```python
from build123d import *

# Parameters (mm, degrees)
F1_DEPTH = 29
F3_DEPTH = 21
F5_D     = 5
F6_D     = 5
F7_D     = 5
F7_DEPTH = 10
F7_TIP   = 1.5021515476
F9_D     = 11.2


with BuildPart() as f1:
    # F0 (on Right) → F1 (new body, symmetric)
    with BuildSketch(Plane.YZ):
        Polygon((-22.1, 20), (-25, 20), (-25, -20), (25, -20), (25, 20), (22.1, 20), (0, -2.1), align=None)
    extrude(amount=F1_DEPTH, both=True)

    # F2 (on Right) → F3 (cut, symmetric)
    with BuildSketch(Plane.YZ):
        Polygon((7, -20), (25, -20), (25, -2), align=None)
    extrude(amount=F3_DEPTH, both=True, mode=Mode.SUBTRACT)

    # F5 (through all)
    with Locations(Plane(origin=(-29, 0, 0), x_dir=(0, -1, 0), z_dir=(-1, 0, 0))):
        with Locations((-19, -14), (19, -14)):
            Hole(F5_D / 2)

    # F6 (through all)
    with Locations(Plane(origin=(-29, 0, 0), x_dir=(0, -1, 0), z_dir=(-1, 0, 0))):
        with Locations((-19, 6), (19, 6)):
            Hole(F6_D / 2)

    # F7
    with Locations(Plane(origin=(-29, 0, 0), x_dir=(0, -1, 0), z_dir=(-1, 0, 0))):
        with Locations((-19, -4), (19, -4)):
            Hole(F7_D / 2, depth=F7_DEPTH)
            with Locations((0, 0, -(F7_DEPTH + F7_TIP / 2))):  # 118° drill point
                Cone(0, F7_D / 2, F7_TIP, mode=Mode.SUBTRACT)

    # F9 (through all)
    with Locations(Plane(origin=(0, 13.5, -13.5), x_dir=(-1, 0, 0), z_dir=(0, 0.7071067812, -0.7071067812))):
        with Locations((-10.5, 4.5150757595), (10.5, 4.5150757595)):
            Hole(F9_D / 2)


solid = f1.part
```
Could you check a few things on this model? Use its own coordinates, in mm. A direction names the side the tool comes from. Coordinates: 2 decimals unless noted, no trailing zeros. Write each loop counter-clockwise with the first axis right and the second up, starting at its lowest first coordinate (ties: lowest second). Pieces come first, ordered by that corner, then holes. Notation, with made-up numbers: (76, 74.25) -> (117, 74.25) arc R24 cw to (117, 105.25) -> close; hole circle Ø6 at (-26.75, 4.5). An arc over 180 degrees is marked (long way). Write item = value, one per line. Start each with the question number.
(1) We'd pull the mould along Z, two halves only. Please class faces 5 (the face through (0, 16, -11)), 6 (the face through (0.4, 11.2, 9.1)), 7 (the face through (0.4, -21.5, 6.1)): released by +Z, released by -Z, zero draft, split by the parting line, or undercut.
(2) Which directions (+Z, -Z, +X, -X, +Y, -Y) give clear straight access to the entire face, cutting with the end or side of a thin tool? Please do faces 1 (the face through (-23.9, 16.5, -3.9)), 2 (the face through (0.4, -10.9, 8.8)), 3 (the face through (21, 20, -17)), 4 (the face through (0.4, -21.5, -13.9)).
(3) I want a section at A-A (x = 10). Please give me the cut outline in (y, z), plus the area to 3 significant figures.
(4) I need wall thicknesses on line 1 (Z direction, x = -22.75, y = 19); line 2 (Z direction, x = 10, y = -19); line 3 (X direction, y = 12, z = -1). Which ranges of each line are inside material? Lowest first, please. Write a range as [from, to].
(5) I want a section at B-B (y = -14). Please give me the cut outline in (x, z), plus the area to 3 significant figures.
(6) Will these pins go through, and if not, where does the flat tip stop? pin 1 (8 mm diameter, centred on y = -19, z = -4, fed in from -X); pin 2 (8 mm diameter, centred on x = 0.5, y = -5.5, fed in from +Z); pin 3 (10 mm diameter, centred on x = 4, y = -2, fed in from +Z); pin 4 (8 mm diameter, centred on x = -21.5, y = 6.5, fed in from +Z).
(7) I want a section at D-D (y = 12). Give the number of separate pieces and of enclosed holes in the cut face, plus the area to 3 significant figures.
(8) I want a section at C-C (y = -6.5). Please give me the cut outline in (x, z), plus the area to 3 significant figures.
Result set:
q1.face_5 = released by -Z
q1.face_6 = released by +Z
q1.face_7 = undercut
q2.face_1 = -X
q2.face_2 = +Z, +X, -X
q2.face_3 = -Z, +Y
q2.face_4 = +X, -X
q3.outline = (-25, -20) -> (7, -20) -> (12.75, -14.25) -> (0.3, -1.8) -> (0, -2.1) -> (-22.1, 20) -> (-25, 20) -> close; (8.19, 6.09) -> (20.64, -6.36) -> (25, -2) -> (25, 20) -> (22.1, 20) -> close; hole circle Ø5 at (-19, -14); hole circle Ø5 at (-19, 6); hole circle Ø5 at (19, 6)
q3.area = 1,090 mm2
q4.line_1 = [-20, -16.5], [-11.5, -6.5], [-1.5, 3.5], [8.5, 16.9]
q4.line_2 = [-20, -16.5], [-11.5, 3.5], [8.5, 16.9]
q4.line_3 = [-29, -15.05], [-5.95, 5.95], [15.05, 29]
q5.outline = (-29, -20) -> (29, -20) -> (29, 11.9) -> (-29, 11.9) -> close
q5.area = 1,850 mm2
q6.pin_1 = -29
q6.pin_2 = 7.4
q6.pin_3 = 4.9
q6.pin_4 = 8.4
q7.separate_pieces = 1
q7.enclosed_holes = 2
q7.area = 1,250 mm2
q8.outline = (-29, -20) -> (29, -20) -> (29, 4.4) -> (-29, 4.4) -> close
q8.area = 1,420 mm2
